Can you work these out from the model? Positions are in its coordinate system, mm. Give positions to 0.01 mm unless a question says otherwise; leave off trailing zeros. Loops run counter-clockwise (first coordinate to the right, second up) from the corner with the lowest first, then second, coordinate; pieces in that order, holes last. Notation, with made-up numbers: (85.5, 71.25) -> (129.5, 71.25) arc R24 ccw to (129.5, 105.25) -> close; hole circle Ø7 at (35.25, -37). An arc over 180 degrees is marked (long way). One line per question, with ' | ' between items.
from build123d import *

# Parameters (mm, degrees)
SKETCH1_R           = 61
SKETCH1_R_2         = 2.5
BOSS_EXTRUDE1_DEPTH = 8


with BuildPart() as part:
    # Sketch1 → Boss-Extrude1 (new body)
    with BuildSketch(Plane(origin=(0, 0, 0), x_dir=(-1, 0, 0), z_dir=(0, 0, 1))):
        with Locations(Location((0, -1, 0), (0, 0, 180))):
            Circle(SKETCH1_R)
        with Locations(Location((0, 54, 0), (0, 0, 180))):
            Circle(SKETCH1_R_2, mode=Mode.SUBTRACT)
        with Locations(Location((46.765371804, 27, 0), (0, 0, 180))):
            Circle(SKETCH1_R_2, mode=Mode.SUBTRACT)
        with Locations(Location((46.765371804, -27, 0), (0, 0, 180))):
            Circle(SKETCH1_R_2, mode=Mode.SUBTRACT)
        with Locations(Location((0, -54, 0), (0, 0, 180))):
            Circle(SKETCH1_R_2, mode=Mode.SUBTRACT)
        with Locations(Location((-46.765371804, -27, 0), (0, 0, 180))):
            Circle(SKETCH1_R_2, mode=Mode.SUBTRACT)
        with Locations(Location((-46.765371804, 27, 0), (0, 0, 180))):
            Circle(SKETCH1_R_2, mode=Mode.SUBTRACT)
    extrude(amount=BOSS_EXTRUDE1_DEPTH)


solid = part.part
Q1. If I drill on probe 1 along Y at (x, z) = (0, 2.5); probe 2 along Y at (x, z) = (-2, 7.75); probe 3 along X at (y, z) = (-52.5, 1.75), over which ranges is the centre line in solid material (lowest first)? Write a range as from..to.
Entries:
probe 1: -60..-56.5, -51.5..51.5, 56.5..62 | probe 2: -59.97..-55.5, -52.5..52.5, 55.5..61.97 | probe 3: -29.3..-2, 2..29.3
Q2. For pin 1 Ø8 at (x, y) = (46.77, 27) entering from +Z; pin 2 Ø1 at (y, z) = (9, 1) entering from +X; pin 3 Ø2 at (y, z) = (10.5, 2.5) entering from -X; pin 4 Ø3 at (x, z) = (-37, 1.5) entering from +Y, each with a flat end and sliding along its axis, tell me the tip position at first contact or that it passes through.
Entries:
pin 1: z = 8 | pin 2: x = 60.54 | pin 3: x = -60.4 | pin 4: y = 50.61
Q3. If we section it at D-D (y = -27): Write out the boundary of the cut face in (x, z).
Entries:
outline: (-54.19, 0) -> (-49.27, 0) -> (-49.27, 8) -> (-54.19, 8) -> close; (-44.27, 0) -> (44.27, 0) -> (44.27, 8) -> (-44.27, 8) -> close; (49.27, 0) -> (54.19, 0) -> (54.19, 8) -> (49.27, 8) -> close
Q4. If we section it at B-B (z = 4.5): Write out the boundary of the cut face in (x, y), plus the area to 3 significant figures.
Entries:
outline: circle Ø122 at (0, 1); hole circle Ø5 at (-46.77, -27); hole circle Ø5 at (-46.77, 27); hole circle Ø5 at (0, -54); hole circle Ø5 at (0, 54); hole circle Ø5 at (46.77, -27); hole circle Ø5 at (46.77, 27) | area: 11,600 mm²
Q5. If we section it at A-A (x = 0): Write out the boundary of the cut face in (y, z).
Entries:
outline: (-60, 0) -> (-56.5, 0) -> (-56.5, 8) -> (-60, 8) -> close; (-51.5, 0) -> (51.5, 0) -> (51.5, 8) -> (-51.5, 8) -> close; (56.5, 0) -> (62, 0) -> (62, 8) -> (56.5, 8) -> close
Q6. If we mould it in two halves opening along X, with no side actions, what happens to faces 1 (the face through (48.109, 29.108, 3.944)), 2 (the face through (-1, 2, 0)), 3 (the face through (-13.22, -58.55, 3.94))? For each: pulls with the +X half, pulls with the -X half, needs draft (parallel to the pull), parting line crosses it, or undercut.
Entries:
face 1: undercut | face 2: needs draft | face 3: parting line crosses it
Q7. If we section it at C-C (y = 54): Write out the boundary of the cut face in (x, z).
Entries:
outline: (-30.2, 0) -> (-2.5, 0) -> (-2.5, 8) -> (-30.2, 8) -> close; (2.5, 0) -> (30.2, 0) -> (30.2, 8) -> (2.5, 8) -> close
